Can you work these out from the drawing? Everything is in mm from the part's minimum corner. A direction names the side the tool comes from. Coordinates: 2 decimals unless noted, no trailing zeros. Order: outer loops, then holes, each group sorted by start corner. A loop starts at its lowest first (then second) coordinate and runs counter-clockwise, first axis right, second up. Notation, with made-up numbers: (0.5, 24) -> (32.5, 24) arc R28 cw to (32.5, 44) -> close; hole circle Ø10 at (5, 66.5). An arc over 180 degrees is marked (long way). Use a Markdown table: item, result. Add a question column.
1) Will these pins go through, and if not, where does the flat tip stop? pin 1 Ø6 at (y, z) = (13, 6) entering from -X; pin 2 Ø2 at (x, z) = (5, 6) entering from +Y (1 decimal).
2) If we section it at C-C (y = 14): Write out the boundary of the cut face in (x, z) (1 decimal).
3) If we section it at D-D (x = 10): Write out the boundary of the cut face in (y, z), plus the area to 3 significant figures.
4) Thinking about a two-plate mould opening in X: for the marked faces 1, 2, 3 and 4, which applies, +X half, -X half, draft (parallel to the pull), parting line (faces both ways), or undercut?
5) If we section it at A-A (y = 6.25): Write out the boundary of the cut face in (x, z), plus the area to 3 significant figures.
6) If I drill on L1, parallel to X at y = 8.25, z = 1.75; L2, parallel to Y at x = 1.25, z = 6; L3, parallel to Z at x = 18.75, y = 14.5, over which ranges is the centre line in solid material (lowest first)? Write a range as [from, to].
7) Which directions (+Z, -Z, +X, -X, +Y, -Y) give clear straight access to the entire face, cutting with the end or side of a thin tool? Please do the marked faces 5 and 6.
8) If we section it at B-B (z = 8.75): Give the number of separate pieces and of enclosed holes in the cut face.
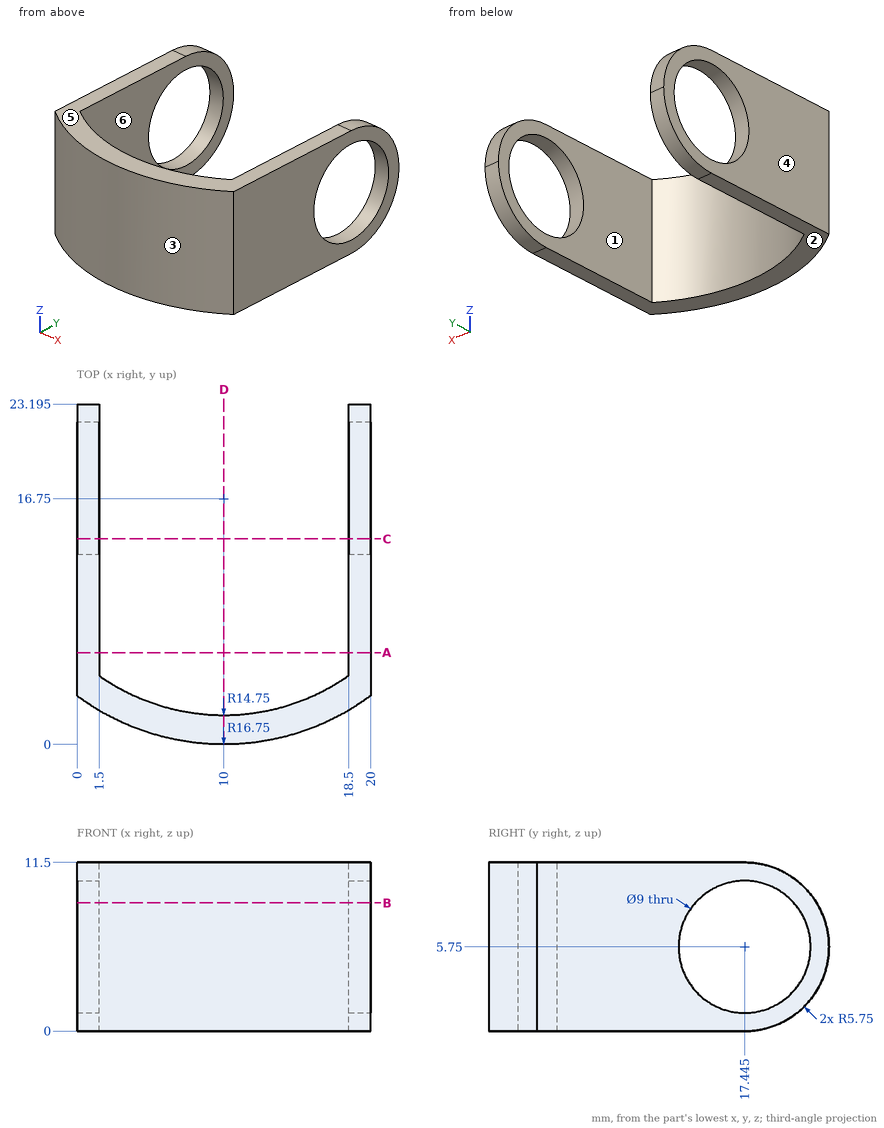
Answer sheet:
| question | item | result |
|---|---|---|
| 1 | pin 1 | x = 0 |
| 1 | pin 2 | y = 3.3 |
| 2 | outline | (0, 0) -> (1.5, 0) -> (1.5, 2.9) -> (0, 2.9) -> close; (0, 8.6) -> (1.5, 8.6) -> (1.5, 11.5) -> (0, 11.5) -> close; (18.5, 0) -> (20, 0) -> (20, 2.9) -> (18.5, 2.9) -> close; (18.5, 8.6) -> (20, 8.6) -> (20, 11.5) -> (18.5, 11.5) -> close |
| 3 | outline | (0, 0) -> (2, 0) -> (2, 11.5) -> (0, 11.5) -> close |
| 3 | area | 23.0 mm2 |
| 4 | face 1 | undercut |
| 4 | face 2 | draft |
| 4 | face 3 | parting line |
| 4 | face 4 | -X half |
| 5 | outline | (0, 0) -> (1.5, 0) -> (1.5, 11.5) -> (0, 11.5) -> close; (18.5, 0) -> (20, 0) -> (20, 11.5) -> (18.5, 11.5) -> close |
| 5 | area | 34.5 mm2 |
| 6 | L1 | [0, 1.5], [18.5, 20] |
| 6 | L2 | [2.47, 12.95], [21.94, 23.19] |
| 6 | L3 | [0, 2.35], [9.15, 11.5] |
| 7 | face 5 | +Z, +X, -X, +Y, -Y |
| 7 | face 6 | +Z, -Z, +Y |
| 8 | separate pieces | 3 |
| 8 | enclosed holes | 0 |
